Work out the finished part from the listing and answer in its coordinate system (mm). A direction names the side the tool comes from. Round coordinates to 2 decimals unless told otherwise and drop trailing zeros. Loops run counter-clockwise (first coordinate to the right, second up) from the corner with the lowest first, then second, coordinate; pieces in that order, holes last. Notation, with made-up numbers: (40.25, 89) - (96.25, 89) arc R37 cw to (96.25, 126) - close; hole circle Ø10 at (-18.5, 58). An arc over 180 degrees is marked (long way). Return JSON: item names as keys, results as strings.
from build123d import *

# Parameters (mm, degrees)
BOSS_EXTRU_1_DEPTH      = 20
D_GAGEMENT_M51_D        = 5.3
D_GAGEMENT_M51_DEPTH    = 45
D_GAGEMENT_M51_TIP      = 1.59228064
ESQUISSE5_R             = 4.5
ENL_V_MAT_EXTRU_1_DEPTH = 20
ENL_V_MAT_EXTRU_2_DEPTH = 20


with BuildPart() as part:
    # Esquisse1 → Boss.-Extru.1 (new body)
    with BuildSketch(Plane.XY):
        with BuildLine():
            Line((-28, 0), (28, 0))
            ThreePointArc((28, 0), (0, -28), (-28, 0))
        make_face()
    extrude(amount=-BOSS_EXTRU_1_DEPTH)

    # Esquisse2 → Enlèvement de matière-Révolution1 (revolve, cut)
    with BuildSketch(Plane(origin=(0, 0, 0), x_dir=(1, 0, 0), z_dir=(0, 1, 0))):
        Polygon((12.15, 24), (12.15, 25), (0, 25), (0, 0), (10, 0), (9, 7.3), (9, 11), (7, 11), (7, 17), (9, 17), (9, 20), (7.25, 20), (7.25, 21.5), (9, 21.5), (9, 22.5), (7.25, 22.5), (7.25, 24), align=None)
    revolve(axis=Axis((0, 0, 0), (0, 0, -1)), mode=Mode.SUBTRACT)

    # Dégagement M51
    with Locations(Plane(origin=(0, 0, 0), x_dir=(1, 0, 0), z_dir=(0, 1, 0))):
        with Locations((-13, 10), (13, 10)):
            Hole(D_GAGEMENT_M51_D / 2, depth=D_GAGEMENT_M51_DEPTH)
            with Locations((0, 0, -(D_GAGEMENT_M51_DEPTH + D_GAGEMENT_M51_TIP / 2))):  # 118° drill point
                Cone(0, D_GAGEMENT_M51_D / 2, D_GAGEMENT_M51_TIP, mode=Mode.SUBTRACT)

    # Esquisse5 → Enlèv. mat.-Extru.1 (cut)
    with BuildSketch(Plane(origin=(0, -28, 0), x_dir=(0, 0, 1), z_dir=(0, -1, 0))):
        with Locations(Location((-10, 13, 0), (0, 0, 180))):
            Circle(ESQUISSE5_R)
        with Locations(Location((-10, -13, 0), (0, 0, 180))):
            Circle(ESQUISSE5_R)
    extrude(amount=-ENL_V_MAT_EXTRU_1_DEPTH, mode=Mode.SUBTRACT)

    # Esquisse6 → Enlèv. mat.-Extru.2 (cut)
    with BuildSketch(Plane.XY):
        with BuildLine():
            Line((-23.643180835, -15), (23.643180835, -15))
            ThreePointArc((23.643180835, -15), (0, -28), (-23.643180835, -15))
        make_face()
    extrude(amount=-ENL_V_MAT_EXTRU_2_DEPTH, mode=Mode.SUBTRACT)


solid = part.part
1) Flat-ended cylindrical pins translate along their axes: pin 1 (7 mm diameter, centred on x = 13, z = -10, fed in from -Y); pin 2 (4 mm diameter, centred on y = -10, z = -5.5, fed in from +X); pin 3 (6 mm diameter, centred on y = -9, z = -2.5, fed in from -X). Find the tip coordinate at first contact, or state that the pin passes through.
Verdict:
{"pin 1": "stops at y = -8", "pin 2": "stops at x = 26.83", "pin 3": "stops at x = -27.35"}
2) Section C-C (x = 0) is taken. Give the vertices of the cut face in (y, z).
Verdict:
{"outline": "(-15, -20) - (-9, -20) - (-9, -17) - (-7, -17) - (-7, -11) - (-9, -11) - (-9, -7.3) - (-10, 0) - (-15, 0) - close"}
3) Section A-A (x = 13) is taken. Give the vertices of the cut face in (y, z), and give its area (3 significant figures).
Verdict:
{"outline": "(-15, -20) - (0, -20) - (0, -12.65) - (-8, -12.65) - (-8, -14.5) - (-15, -14.5) - close; (-15, -5.5) - (-8, -5.5) - (-8, -7.35) - (0, -7.35) - (0, 0) - (-15, 0) - close", "area": "195 mm2"}
4) Find the intervals of material crossed by L1, parallel to X at y = -4.25, z = -10; L2, parallel to X at y = -13.5, z = -10; L3, parallel to Z at x = -13, y = -1.25, in increasing order.
Verdict:
{"L1": "x = -27.68 to -15.65, -10.35 to -7.93, 7.93 to 10.35, 15.65 to 27.68", "L2": "x = -24.53 to -17.5, -8.5 to 8.5, 17.5 to 24.53", "L3": "z = -20 to -12.65, -7.35 to 0"}
5) Section D-D (z = -14) is taken. Give the vertices of the cut face in (x, y).
Verdict:
{"outline": "(-28, 0) arc R28 ccw to (-23.64, -15) - (-15.06, -15) - (-15.06, -8) - (-10.94, -8) - (-10.94, -15) - (10.94, -15) - (10.94, -8) - (15.06, -8) - (15.06, -15) - (23.64, -15) arc R28 ccw to (28, 0) - (7, 0) arc R7 cw to (-7, 0) - close"}
6) Section B-B (y = -5.25) is taken. Count the separate pieces of the cut face and the enclosed holes in it, and give its area (3 significant figures).
Verdict:
{"separate pieces": "2", "enclosed holes": "2", "area": "787 mm2"}
7) A tool of negligible diameter and unlimited length cuts with its end or side. For faces 5 (the flat face through (11, -8, -12)), 6 (the flat face through (17, 0, -10)), 7 (the cylindrical face through (0, -9, -19)), 8 (the cylindrical face through (0, -9, -9)), 9 (the cylindrical face through (26.92, -7.7, -9.86)), from which of +Z, -Z, +X, -X, +Y, -Y can it reach the whole face along a straight path? Write none if from no direction.
Verdict:
{"face 5": "-Y", "face 6": "+Z, -Z, +X, -X, +Y", "face 7": "-Z, +Y", "face 8": "+Z, +Y", "face 9": "+Z, -Z, +X, -Y"}
8) Determine the mould class of faces 1 (the flat face through (-0.6, -7.2, -17)), 2 (the flat face through (0, -11, 0)), 3 (the cylindrical face through (-11.648, -11.549, -14.292)), 4 (the cylindrical face through (-26.858, -7.916, -9.86)) for opening direction Z: pulls with the +Z half, pulls with the -Z half, needs draft (parallel to the pull), parting line crosses it, or undercut.
Verdict:
{"face 1": "pulls with the -Z half", "face 2": "pulls with the +Z half", "face 3": "undercut", "face 4": "needs draft"}
